```python
from build123d import *

# Parameters (mm, degrees)
EXTRUDE_1_DEPTH     = 15
CUT_EXTRUDE_1_DEPTH = 5
SKETCH_3_R          = 1.6
SKETCH_3_W          = 5
SKETCH_3_H          = 5
CUT_EXTRUDE_2_DEPTH = 22
FILLET_1_R          = 2


with BuildPart() as part:
    # 草图1 → 凸台-拉伸1 (new body)
    with BuildSketch(Plane.XY):
        with BuildLine():
            Line((24.185160084, -7.016301696), (24.496510845, 5.979969335))
            ThreePointArc((24.496510845, 5.979969335), (23.944762934, 7.407806858), (22.544984649, 8.027295764))
            Line((22.544984649, 8.027295764), (-13.444688974, 8.889497871))
            Line((-13.444688974, 8.889497871), (-13.265063535, 16.387346543))
            Line((-13.265063535, 16.387346543), (-18.263629316, 16.507096835))
            ThreePointArc((-18.263629316, 16.507096835), (-21.833223125, 15.127727058), (-23.38194539, 11.628281347))
            Line((-23.38194539, 11.628281347), (-23.908846678, -10.36540809))
            ThreePointArc((-23.908846678, -10.36540809), (-22.5294769, -13.935001898), (-19.030031189, -15.483724163))
            Line((-19.030031189, -15.483724163), (-14.031465408, -15.603474456))
            Line((-14.031465408, -15.603474456), (-13.851839969, -8.105625784))
            Line((-13.851839969, -8.105625784), (22.137833654, -8.967827891))
            ThreePointArc((22.137833654, -8.967827891), (23.565671178, -8.41607998), (24.185160084, -7.016301696))
        make_face()
        with BuildLine():
            ThreePointArc((-16.75044735, -12.037331753), (-18.893602347, -9.788969482), (-21.141964619, -11.93212448))
            ThreePointArc((-21.141964619, -11.93212448), (-18.998809621, -14.180486751), (-16.75044735, -12.037331753))
        make_face(mode=Mode.SUBTRACT)
        with BuildLine():
            ThreePointArc((-16.04728092, -4.552025517), (-18.701434473, -1.76757982), (-21.48588017, -4.421733373))
            ThreePointArc((-21.48588017, -4.421733373), (-18.831726617, -7.20617907), (-16.04728092, -4.552025517))
        make_face(mode=Mode.SUBTRACT)
        with BuildLine():
            ThreePointArc((-15.807780335, 5.445106045), (-18.461933888, 8.229551742), (-21.246379585, 5.575398189))
            ThreePointArc((-21.246379585, 5.575398189), (-18.592226032, 2.790952492), (-15.807780335, 5.445106045))
        make_face(mode=Mode.SUBTRACT)
        with BuildLine():
            ThreePointArc((-16.151695887, 12.955497152), (-18.294850884, 15.203859423), (-20.543213156, 13.060704426))
            ThreePointArc((-20.543213156, 13.060704426), (-18.400058158, 10.812342154), (-16.151695887, 12.955497152))
        make_face(mode=Mode.SUBTRACT)
    extrude(amount=-EXTRUDE_1_DEPTH)

    # 草图2 → 切除-拉伸1 (cut)
    with BuildSketch(Plane(origin=(0, 0, -15), x_dir=(-1, 0, 0), z_dir=(0, 0, -1))):
        Polygon((13.444688974, 8.889497871), (13.851839969, -8.105625784), (-33.415838559, -15.121344773), (-27.379501609, 15.743180277), align=None)
    extrude(amount=-CUT_EXTRUDE_1_DEPTH, mode=Mode.SUBTRACT)

    # 草图3 → 切除-拉伸2 (cut)
    with BuildSketch(Plane(origin=(0.205130979, 8.562490084, 0), x_dir=(0.9997131562086496, -0.02395005852477245, 0), z_dir=(0.02395005852477245, 0.9997131562086496, 0))):
        with Locations(Location((21.846263557, 5, 0), (0, 0, 288.209956864))):
            Circle(SKETCH_3_R)
        with Locations(Location((-8.153736443, 5, 0), (0, 0, 180))):
            Circle(SKETCH_3_R)
        with Locations((9.846263557, 7.5)):
            Rectangle(SKETCH_3_W, SKETCH_3_H)
    extrude(amount=-CUT_EXTRUDE_2_DEPTH, mode=Mode.SUBTRACT)

    # 圆角1
    fillet_1_edges = [part.edges().sort_by_distance(p)[0] for p in [
        (7.142136311, -8.608577013, -7.5),
        (7.549287306, 8.386546642, -7.5),
    ]]
    fillet(fillet_1_edges, radius=FILLET_1_R)


solid = part.part
```
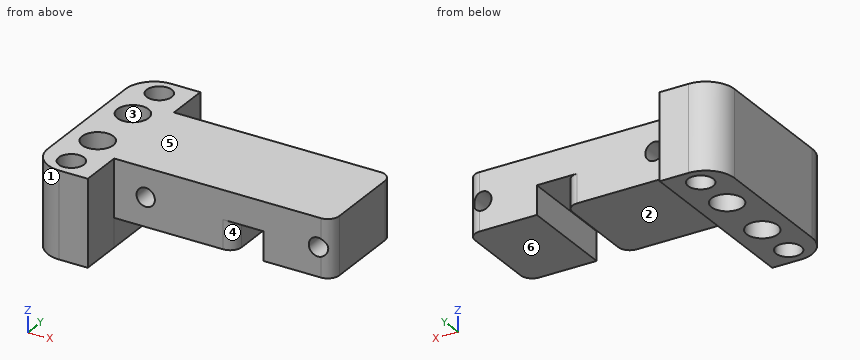
Verification items for the finished model (mm, model axes). Face numbers are marked on the shaded views. A direction names the side the tool comes from. Coordinates: 2 decimals unless noted, no trailing zeros. Loops run counter-clockwise (first coordinate to the right, second up) from the corner with the lowest first, then second, coordinate; pieces in that order, holes last. Notation, with made-up numbers: (68, 42) - (121, 42) arc R27 ccw to (121, 81) - close; hole circle Ø10 at (-5, -21.5). An arc over 180 degrees is marked (long way). Return JSON: item names as keys, results as strings.
1. Section check B-B, the plane y = -11. Record the boundary of the cut face in (x, z), then the cut area to 3 significant figures.
Established:
{"outline": "(-23.88, -15) - (-20.91, -15) - (-20.91, 0) - (-23.88, 0) - close; (-16.98, -15) - (-13.92, -15) - (-13.92, 0) - (-16.98, 0) - close", "area": "90.5 mm2"}
2. Mould release check, pull along X, two halves, no side actions. Record for the marked faces 1, 2 and 3: +X half, -X half, draft (parallel to the pull), parting line (faces both ways), or undercut.
Established:
{"face 1": "-X half", "face 2": "draft", "face 3": "undercut"}
3. Section check C-C, the plane z = -1.25. Record the boundary of the cut face in (x, y), then the cut area to 3 significant figures.
Established:
{"outline": "(-23.91, -10.37) arc R5 ccw to (-19.03, -15.48) - (-14.03, -15.6) - (-13.85, -8.11) - (22.14, -8.97) arc R2 ccw to (24.19, -7.02) - (24.5, 5.98) arc R2 ccw to (22.54, 8.03) - (-13.44, 8.89) - (-13.27, 16.39) - (-18.26, 16.51) arc R5 ccw to (-23.38, 11.63) - close; hole circle Ø5.44 at (-18.77, -4.49); hole circle Ø5.44 at (-18.53, 5.51); hole circle Ø4.39 at (-18.95, -11.98); hole circle Ø4.39 at (-18.35, 13.01)", "area": "877 mm2"}
4. Go/stop test with flat-tipped pins: pin 1 (4 mm diameter, centred on x = 19, z = -13, fed in from +Y); pin 2 (14 mm diameter, centred on x = 0, y = -3, fed in from -Z); pin 3 (5 mm diameter, centred on x = 12.5, y = -3, fed in from +Z); pin 4 (2 mm diameter, centred on x = 9.5, y = 3.5, fed in from -Z). Record where each tip stops, or that it passes through.
Established:
{"pin 1": "passes through", "pin 2": "stops at z = -10", "pin 3": "stops at z = 0", "pin 4": "stops at z = -5"}
5. Tool access check on the marked faces 4, 5 and 6. Record the directions out of +Z, -Z, +X, -X, +Y, -Y that give a thin tool (end or side, any length) a straight path to the whole face; none if there is none.
Established:
{"face 4": "-Z, -Y", "face 5": "+Z, +X, -X, +Y, -Y", "face 6": "-Z, +X, +Y, -Y"}
6. Section check D-D, the plane y = -6. Count the separate pieces of the cut face and the enclosed holes in it, then the cut area to 3 significant figures.
Established:
{"separate pieces": "2", "enclosed holes": "2", "area": "421 mm2"}
7. Section check A-A, the plane z = -5.75. Record the boundary of the cut face in (x, y).
Established:
{"outline": "(-23.91, -10.37) arc R5 ccw to (-19.03, -15.48) - (-14.03, -15.6) - (-13.85, -8.11) - (-9.77, -8.2) - (-9.36, 8.79) - (-13.44, 8.89) - (-13.27, 16.39) - (-18.26, 16.51) arc R5 ccw to (-23.38, 11.63) - close; (-6.94, -8.27) - (5.14, -8.56) arc R2 ccw to (7.19, -6.61) - (7.5, 6.39) arc R2 ccw to (5.55, 8.43) - (-6.53, 8.72) - close; (12.14, -8.73) - (20.23, -8.92) - (20.63, 8.07) - (12.55, 8.27) - close; (23.06, -8.77) arc R2 ccw to (24.19, -7.02) - (24.5, 5.98) arc R2 ccw to (23.45, 7.78) - close; hole circle Ø5.44 at (-18.77, -4.49); hole circle Ø5.44 at (-18.53, 5.51); hole circle Ø4.39 at (-18.95, -11.98); hole circle Ø4.39 at (-18.35, 13.01)"}
8. Thickness scan on L1, parallel to Y at x = -19.5, z = -2.25; L2, parallel to Z at x = 13, y = 7; L3, parallel to X at y = 13, z = -5.5. Record the ranges inside material, lowest first.
Established:
{"L1": "y = -15.45 to -14.11, -9.86 to -7.11, -1.87 to 2.97, 8.05 to 11.14, 14.88 to 16.38", "L2": "z = -10 to 0", "L3": "x = -23.16 to -20.54, -16.15 to -13.35"}
